from build123d import *

# Parameters (mm, degrees)
SKETCH1_W                = 304.8
SKETCH1_H                = 304.8
BOSS_EXTRUDE2_DEPTH      = 304.8
SHELL1_T                 = -12.7
SKETCH2_R                = 3.877794573
BOSS_EXTRUDE3_DEPTH      = 6
M2_5X0_45_TAPPED_HOLE3_D = 2.05


with BuildPart() as part:
    # Sketch1 → Boss-Extrude2 (new body)
    with BuildSketch(Plane.XY):
        with Locations((141.322807232, 102.754701441)):
            Rectangle(SKETCH1_W, SKETCH1_H)
    extrude(amount=BOSS_EXTRUDE2_DEPTH)

    # Shell1
    shell1_openings = [part.faces().sort_by_distance(p)[0] for p in [
        (141.322807232, 255.154701441, 152.4),
    ]]
    offset(amount=SHELL1_T, openings=shell1_openings, kind=Kind.INTERSECTION)

    # Sketch2 → Boss-Extrude3 (add)
    with BuildSketch(Plane(origin=(0, -36.945298559, 0), x_dir=(1, 0, 0), z_dir=(0, 1, 0))):
        with Locations(Location((115.822807232, -131.4, 0), (0, 0, 270))):
            Circle(SKETCH2_R)
        with BuildLine():
            Line((168.492325351, -127.9), (165.153289112, -127.9))
            ThreePointArc((165.153289112, -127.9), (164.080792393, -134.142014839), (170.322807232, -133.069518119))
            Line((170.322807232, -133.069518119), (170.322807232, -129.730481881))
            ThreePointArc((170.322807232, -129.730481881), (169.56482207, -128.657985161), (168.492325351, -127.9))
        make_face()
        with BuildLine():
            ThreePointArc((117.492325351, -176.9), (118.56482207, -170.657985161), (112.322807232, -171.730481881))
            Line((112.322807232, -171.730481881), (112.322807232, -175.069518119))
            ThreePointArc((112.322807232, -175.069518119), (113.080792393, -176.142014839), (114.153289112, -176.9))
            Line((114.153289112, -176.9), (117.492325351, -176.9))
        make_face()
        with BuildLine():
            Line((170.322807232, -175.069518119), (170.322807232, -171.730481881))
            ThreePointArc((170.322807232, -171.730481881), (164.080792393, -170.657985161), (165.153289112, -176.9))
            Line((165.153289112, -176.9), (168.492325351, -176.9))
            ThreePointArc((168.492325351, -176.9), (169.56482207, -176.142014839), (170.322807232, -175.069518119))
        make_face()
    extrude(amount=BOSS_EXTRUDE3_DEPTH)

    # M2.5x0.45 Tapped Hole3 (through all)
    with Locations(Plane(origin=(0, -30.945298559, 0), x_dir=(1, 0, 0), z_dir=(0, 1, 0))):
        with Locations((115.822807232, -131.4), (166.822807232, -131.4), (166.822807232, -173.4), (115.822807232, -173.4)):
            Hole(M2_5X0_45_TAPPED_HOLE3_D / 2)


solid = part.part
Part model, mm, in its own coordinate system. A direction names the side the tool comes from. Give positions to 0.01 mm unless a question says otherwise; leave off trailing zeros. Order: outer loops, then holes, each group sorted by start corner. A loop starts at its lowest first (then second) coordinate and runs counter-clockwise, first axis right, second up. Notation, with made-up numbers: (33, 5) -> (66, 5) arc R36 ccw to (66, 40) -> close; hole circle Ø1 at (17, 22.5). An arc over 180 degrees is marked (long way). Use one line per item in the form item = value.
(1) Tool access for faces 4 (the face through (139, 111, 292.1)), 5 (the face through (129, 255.155, 298)): list every direction of +Z, -Z, +X, -X, +Y, -Y with a clear straight run to the whole face (end or side of a thin tool).
Solution:
face_4 = +Y
face_5 = +Z, -Z, +X, -X, +Y
(2) Drill centre lines: line 1 (X direction, y = -40.5, z = 131.4); line 2 (Z direction, x = 170, y = 19); line 3 (X direction, y = 64, z = 176). Where is each one in solid material? Low to high. Write a range as from..to.
Solution:
line_1 = -11.08..114.8, 116.85..165.8, 167.85..293.72
line_2 = 0..12.7, 292.1..304.8
line_3 = -11.08..1.62, 281.02..293.72
(3) Saw through at A-A (y = 45). Write the cut outline in (x, z).
Solution:
outline = (-11.08, 0) -> (293.72, 0) -> (293.72, 304.8) -> (-11.08, 304.8) -> close; hole (1.62, 12.7) -> (281.02, 12.7) -> (281.02, 292.1) -> (1.62, 292.1) -> close
(4) Saw through at B-B (z = 100). Write the cut outline in (x, y).
Solution:
outline = (-11.08, -49.65) -> (293.72, -49.65) -> (293.72, 255.15) -> (281.02, 255.15) -> (281.02, -36.95) -> (1.62, -36.95) -> (1.62, 255.15) -> (-11.08, 255.15) -> close
(5) Flat gauge pins, fed straight in: P1, Ø1.5, axis at x = 148.5, z = 53.5, coming from the +Y side; P2, Ø2.5, axis at x = 166.82, z = 131.4, coming from the +Y side. Where does each tip first touch, or does it go through?
Solution:
P1 = -36.95
P2 = -30.95
(6) Saw through at C-C (x = 223.5). Write the cut outline in (y, z).
Solution:
outline = (-49.65, 0) -> (255.15, 0) -> (255.15, 12.7) -> (-36.95, 12.7) -> (-36.95, 292.1) -> (255.15, 292.1) -> (255.15, 304.8) -> (-49.65, 304.8) -> close
(7) Pull direction X, two halves, no side cores. Call faces 1 (the face through (281.023, 107, 150)), 2 (the face through (139, 105, 0)), 3 (the face through (-11.077, 101, 150)): +X half, -X half, draft (parallel to the pull), parting line (faces both ways), or undercut.
Solution:
face_1 = undercut
face_2 = draft
face_3 = -X half
